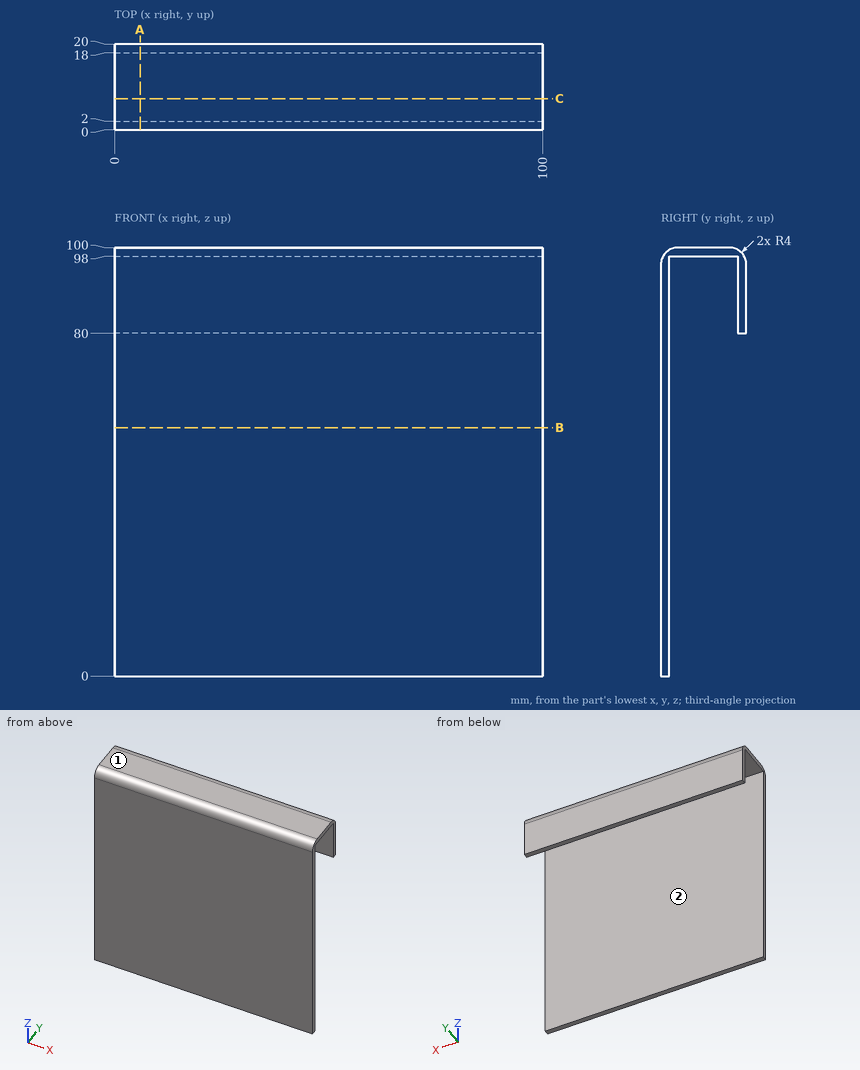
Answer from the drawing. Dimensions are ordinates in mm from the lowest x, y and z of the part. A direction names the side the tool comes from. Round coordinates to 2 decimals unless told otherwise and drop trailing zeros. Loops run counter-clockwise (first coordinate to the right, second up) from the corner with the lowest first, then second, coordinate; pieces in that order, holes last.
1) For the marked faces 1 and 2, determine the directions among +Z, -Z, +X, -X, +Y, -Y from which every point of the face is accessible in a straight line to the end or side of a thin tool.
Outcome:
face 1: +Z, +X, -X, +Y, -Y
face 2: -Z, +X, -X
2) A cutting plane is placed at B-B on z = 58. Determine the outline of the cut face in (x, y).
Outcome:
outline: (0, 0) - (100, 0) - (100, 2) - (0, 2) - close
3) A cutting plane is placed at A-A on x = 6. Determine the outline of the cut face in (y, z).
Outcome:
outline: (0, 0) - (2, 0) - (2, 98) - (18, 98) - (18, 80) - (20, 80) - (20, 96) arc R4 ccw to (16, 100) - (4, 100) arc R4 ccw to (0, 96) - close
4) Given P1, Ø8, axis at x = 29, y = 10.5, coming from the -Z side; P2, Ø2, axis at x = 41, y = 18.5, coming from the -Z side; P3, Ø12, axis at x = 81, z = 66, coming from the +Y side, each flat-ended and moving along its own axis, determine where each tip first touches the part or whether it passes through.
Outcome:
P1: stops at z = 98
P2: stops at z = 80
P3: stops at y = 2
5) Consider line 1 (Y direction, x = 35, z = 84); line 2 (Y direction, x = 14, z = 21.5); line 3 (Z direction, x = 62, y = 8.25). Determine where each line is inside the solid, lowest interval first.
Outcome:
line 1: y = 0 to 2, 18 to 20
line 2: y = 0 to 2
line 3: z = 98 to 100
6) A cutting plane is placed at C-C on y = 7.25. Determine the outline of the cut face in (x, z).
Outcome:
outline: (0, 98) - (100, 98) - (100, 100) - (0, 100) - close
